Part print with two shaded views. Sizes in mm from the minimum x, y, z corner. Give positions to 0.01 mm unless a question says otherwise; leave off trailing zeros. Write each loop counter-clockwise with the first axis right and the second up, starting at its lowest first coordinate (ties: lowest second). Pieces come first, ordered by that corner, then holes. Notation, with made-up numbers: (76, -26) -> (128, -26) arc R11 ccw to (128, -6) -> close; hole circle Ø9 at (42, 64). An arc over 180 degrees is marked (long way). Write item = value, one per line. Start each with the question number.
Q1. Drop flat-ended pins along their axis: P1, Ø4.5, axis at x = 35, z = 5, coming from the +Y side; P2, Ø2, axis at x = 5, z = 5, coming from the +Y side (1 decimal). Give the stop position or say it passes through.
Q2. Saw through at C-C, the plane z = 5. List the corners of the cut face in (x, y).
Q3. Saw through at D-D, the plane x = 5. List the corners of the cut face in (y, z), then the cut area to 3 significant figures.
Q4. Wall check: line 1 (X direction, y = 4, z = 5); line 2 (Y direction, x = 20, z = 2.5); line 3 (X direction, y = 8.25, z = 6). Give the ranges that are in metal, low to high.
Q5. Saw through at A-A, the plane y = 5.6. List the corners of the cut face in (x, z).
Q6. Mould opens along X. For the marked faces 1, 2, 3 and 4 say: pulls with the +X half, pulls with the -X half, needs draft (parallel to the pull), parting line crosses it, or undercut.
Q7. Saw through at B-B, the plane x = 20. List the corners of the cut face in (y, z), then the cut area to 3 significant figures.
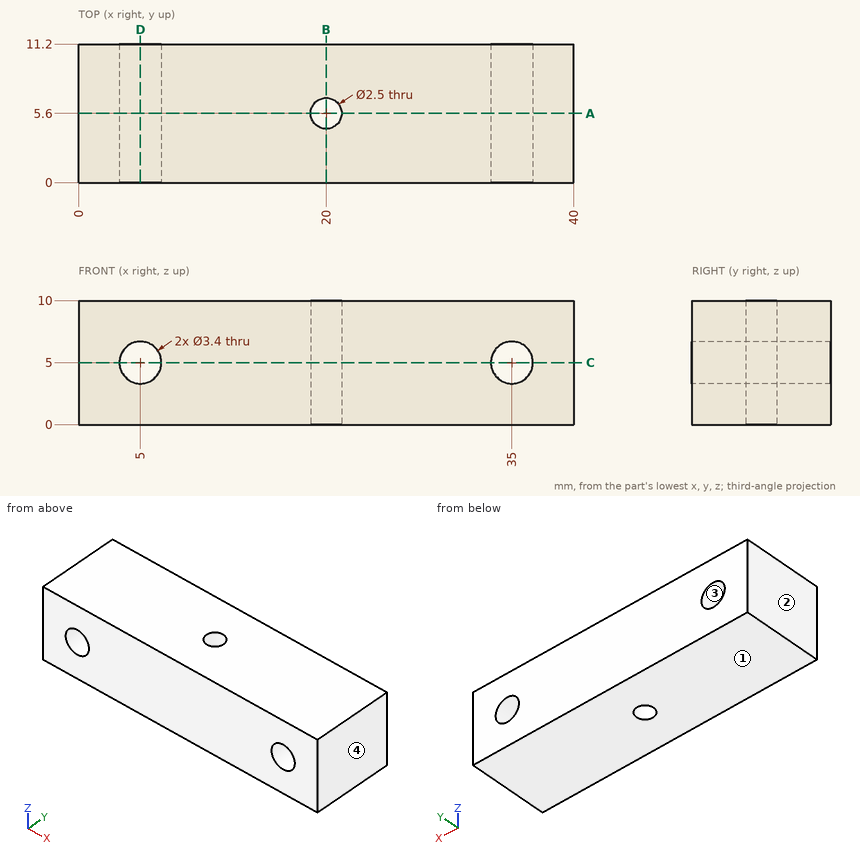
Report:
q1.P1 = 11.2
q1.P2 = through
q2.outline = (0, 0) -> (3.3, 0) -> (3.3, 11.2) -> (0, 11.2) -> close; (6.7, 0) -> (33.3, 0) -> (33.3, 11.2) -> (6.7, 11.2) -> close; (36.7, 0) -> (40, 0) -> (40, 11.2) -> (36.7, 11.2) -> close; hole circle Ø2.5 at (20, 5.6)
q3.outline = (0, 0) -> (11.2, 0) -> (11.2, 3.3) -> (0, 3.3) -> close; (0, 6.7) -> (11.2, 6.7) -> (11.2, 10) -> (0, 10) -> close
q3.area = 73.9 mm2
q4.line_1 = 0 to 3.3, 6.7 to 33.3, 36.7 to 40
q4.line_2 = 0 to 4.35, 6.85 to 11.2
q4.line_3 = 0 to 3.63, 6.37 to 33.63, 36.37 to 40
q5.outline = (0, 0) -> (18.75, 0) -> (18.75, 10) -> (0, 10) -> close; (21.25, 0) -> (40, 0) -> (40, 10) -> (21.25, 10) -> close; hole circle Ø3.4 at (5, 5); hole circle Ø3.4 at (35, 5)
q6.face_1 = needs draft
q6.face_2 = pulls with the -X half
q6.face_3 = undercut
q6.face_4 = pulls with the +X half
q7.outline = (0, 0) -> (4.35, 0) -> (4.35, 10) -> (0, 10) -> close; (6.85, 0) -> (11.2, 0) -> (11.2, 10) -> (6.85, 10) -> close
q7.area = 87.0 mm2
